```python
from build123d import *

# Parameters (mm, degrees)
BOSS_EXTRUDE1_DEPTH = 8.1
BOSS_EXTRUDE2_DEPTH = 11.8
FILLET1_R           = 0.5
FILLET2_R           = 0.5
FILLET4_R           = 0.5


with BuildPart() as part:
    # Sketch8 → Boss-Extrude1 (new body)
    with BuildSketch(Plane(origin=(-2.232753674, 0, 0.665681661), x_dir=(-1, 0, 0), z_dir=(0, -1, 0))):
        Polygon((-24.744344877, -18.877779499), (-23.219344877, -18.877779499), (-23.219344877, -21.527779499), (-24.744344877, -21.527779499), (-24.744344877, -23.052779499), (-27.394344877, -23.052779499), (-27.394344877, -21.527779499), (-28.919344877, -21.527779499), (-28.919344877, -18.877779499), (-27.394344877, -18.877779499), (-27.394344877, -17.352779499), (-24.744344877, -17.352779499), align=None)
        Polygon((-26.694344877, -20.827779499), (-26.694344877, -22.352779499), (-25.444344877, -22.352779499), (-25.444344877, -20.827779499), (-23.919344877, -20.827779499), (-23.919344877, -19.577779499), (-25.444344877, -19.577779499), (-25.444344877, -18.052779499), (-26.694344877, -18.052779499), (-26.694344877, -19.577779499), (-28.219344877, -19.577779499), (-28.219344877, -20.827779499), align=None, mode=Mode.SUBTRACT)
    extrude(amount=BOSS_EXTRUDE1_DEPTH)

    # Sketch9 → Boss-Extrude2 (add)
    with BuildSketch(Plane(origin=(0, 0, 0), x_dir=(-1, 0, 0), z_dir=(0, 1, 0))):
        with BuildLine():
            Line((-20.086591203, 22.61846116), (-20.086591203, 19.11846116))
            ThreePointArc((-20.086591203, 19.11846116), (-23.836591203, 15.36846116), (-27.586591203, 19.11846116))
            Line((-27.586591203, 19.11846116), (-27.586591203, 22.61846116))
            ThreePointArc((-27.586591203, 22.61846116), (-23.836591203, 26.36846116), (-20.086591203, 22.61846116))
        make_face()
    extrude(amount=BOSS_EXTRUDE2_DEPTH)

    # Fillet1
    fillet1_edges = [part.edges().sort_by_distance(p)[0] for p in [
        (22.511591203, -4.05, 19.54346116),
        (20.986591203, -4.05, 19.54346116),
        (20.986591203, -4.05, 22.19346116),
        (22.511591203, -4.05, 22.19346116),
        (22.511591203, -4.05, 23.71846116),
        (25.161591203, -4.05, 23.71846116),
        (25.161591203, -4.05, 22.19346116),
        (26.686591203, -4.05, 22.19346116),
        (26.686591203, -4.05, 19.54346116),
        (25.161591203, -4.05, 19.54346116),
        (25.161591203, -4.05, 18.01846116),
        (22.511591203, -4.05, 18.01846116),
    ]]
    fillet(fillet1_edges, radius=FILLET1_R)

    # Fillet2
    fillet2_edges = [part.edges().sort_by_distance(p)[0] for p in [
        (21.749091203, 0, 19.54346116),
        (20.986591203, 0, 20.86846116),
        (21.749091203, 0, 22.19346116),
        (22.511591203, 0, 22.95596116),
        (23.836591203, 0, 23.71846116),
        (25.161591203, 0, 22.95596116),
        (25.924091203, 0, 22.19346116),
        (26.686591203, 0, 20.86846116),
        (25.924091203, 0, 19.54346116),
        (25.161591203, 0, 18.78096116),
        (23.836591203, 0, 18.01846116),
        (25.308037813, 0, 19.39701455),
        (25.308037813, 0, 22.339907769),
        (22.365144594, 0, 22.339907769),
        (22.365144594, 0, 19.39701455),
        (21.133037813, 0, 19.689907769),
        (21.133037813, 0, 22.04701455),
        (22.658037813, 0, 23.57201455),
        (25.015144594, 0, 23.57201455),
        (26.540144594, 0, 22.04701455),
        (26.540144594, 0, 19.689907769),
        (22.658037813, 0, 18.164907769),
        (25.015144594, 0, 18.164907769),
        (22.511591203, 0, 18.78096116),
    ]]
    fillet(fillet2_edges, radius=FILLET2_R)

    # Fillet4
    fillet4_edges = [part.edges().sort_by_distance(p)[0] for p in [
        (21.749091203, -8.1, 19.54346116),
        (20.986591203, -8.1, 20.86846116),
        (23.836591203, -8.1, 18.01846116),
        (25.161591203, -8.1, 18.78096116),
        (25.924091203, -8.1, 19.54346116),
        (26.686591203, -8.1, 20.86846116),
        (25.924091203, -8.1, 22.19346116),
        (25.161591203, -8.1, 22.95596116),
        (23.836591203, -8.1, 23.71846116),
        (22.511591203, -8.1, 22.95596116),
        (21.749091203, -8.1, 22.19346116),
        (25.015144594, -8.1, 18.164907769),
        (22.658037813, -8.1, 18.164907769),
        (26.540144594, -8.1, 19.689907769),
        (26.540144594, -8.1, 22.04701455),
        (25.015144594, -8.1, 23.57201455),
        (22.658037813, -8.1, 23.57201455),
        (21.133037813, -8.1, 22.04701455),
        (21.133037813, -8.1, 19.689907769),
        (22.365144594, -8.1, 19.39701455),
        (22.365144594, -8.1, 22.339907769),
        (25.308037813, -8.1, 22.339907769),
        (25.308037813, -8.1, 19.39701455),
        (22.511591203, -8.1, 18.78096116),
    ]]
    fillet(fillet4_edges, radius=FILLET4_R)


solid = part.part
```
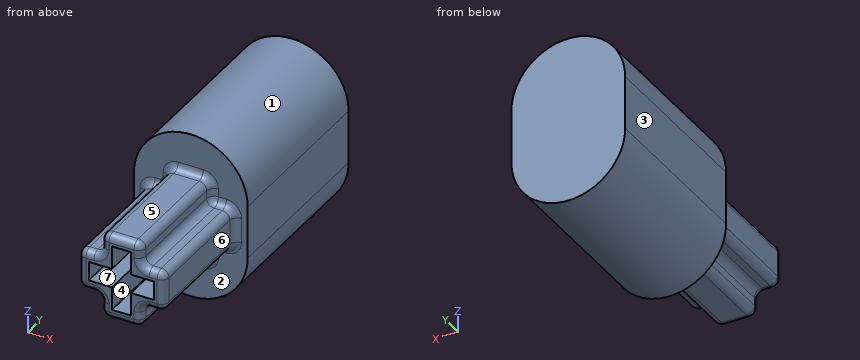
Design review of the part built by this model. Coordinates are the model's own, in mm. Face numbers are marked on the shaded views. A direction names the side the tool comes from. Coordinates: 2 decimals unless noted, no trailing zeros. Order: outer loops, then holes, each group sorted by start corner. A loop starts at its lowest first (then second) coordinate and runs counter-clockwise, first axis right, second up. Notation, with made-up numbers: M 35.25,-17 L 51.25,-17 A15 cw 51.25,8 Z; hole C 20.25,19.5 d1. An arc over 180 degrees is marked long. Answer as a JSON object with one key per item and string values. Group by question number.
1) Tool access review of the marked faces 5, 6 and 7: name each direction out of +Z, -Z, +X, -X, +Y, -Y from which nothing blocks a thin tool from reaching the whole face with its end or side.
2) Add section D-D, the plane z = 25.5. Write out the cut boundary in (x, y), then the cut area to 3 significant figures.
3) Add section C-C, the plane y = 9.5. Write out the cut boundary in (x, z).
4) For pin 1 (0.6 mm diameter, centred on x = 23.5, y = -5, fed in from -Z); pin 2 (0.5 mm diameter, centred on y = -3.5, z = 22, fed in from -X); pin 3 (1.7 mm diameter, centred on x = 25.5, y = -2.5, fed in from +Z), all flat-tipped, find the tip position at first contact; note any pin that passes through.
5) Wall thickness on L1, parallel to Z at x = 23.5, y = -4.75; L2, parallel to Z at x = 25, y = -2.5; L3, parallel to Z at x = 23.75, y = 4.25: over which ranges is each line inside the solid? List them lowest first.
6) Add section B-B, the plane x = 23.5. Write out the cut boundary in (y, z).
7) Mouldability with a two-part tool opening along X and no side actions: class the marked faces 1, 2, 3 and 4 as pulls with the +X half, pulls with the -X half, needs draft (parallel to the pull), parting line crosses it, or undercut.
8) Add section A-A, the plane z = 20.75. Write out the cut boundary in (x, y), then the cut area to 3 significant figures.
Computed values:
{
 "1": {"face 5": "+Z, +X, -X, -Y", "face 6": "+Z, -Z, +X, -Y", "face 7": "-Y"},
 "2": {"outline": "M 21.44,0 L 26.24,0 L 26.24,11.8 L 21.44,11.8 Z", "area": "56.6 mm^2"},
 "3": {"outline": "M 20.09,19.12 A3.75 ccw 27.59,19.12 L 27.59,22.62 A3.75 ccw 20.09,22.62 Z"},
 "4": {"pin 1": "stops at z = 18.02", "pin 2": "stops at x = 20.99", "pin 3": "stops at z = 23.72"},
 "5": {"L1": "z = 18.02 to 18.72, 23.02 to 23.72", "L2": "z = 18.15 to 20.24, 21.49 to 23.59", "L3": "z = 15.37 to 26.37"},
 "6": {"outline": "M -8.1,18.52 A0.5 ccw -7.6,18.02 L -0.5,18.02 A0.5 cw 0,17.52 L 0,15.38 L 11.8,15.38 L 11.8,26.35 L 0,26.35 L 0,24.22 A0.5 cw -0.5,23.72 L -7.6,23.72 A0.5 ccw -8.1,23.22 L -8.1,23.02 L 0,23.02 L 0,18.72 L -8.1,18.72 Z"},
 "7": {"face 1": "parting line crosses it", "face 2": "needs draft", "face 3": "pulls with the -X half", "face 4": "undercut"},
 "8": {"outline": "M 20.09,0 L 20.49,0 A0.5 cw 20.99,-0.5 L 20.99,-7.6 A0.5 ccw 21.49,-8.1 L 21.69,-8.1 L 21.69,0 L 25.99,0 L 25.99,-8.1 L 26.19,-8.1 A0.5 ccw 26.69,-7.6 L 26.69,-0.5 A0.5 cw 27.19,0 L 27.59,0 L 27.59,11.8 L 20.09,11.8 Z", "area": "99.8 mm^2"}
}
